Design review of the part built by this model. Coordinates are the model's own, in mm. Face numbers are marked on the shaded views. A direction names the side the tool comes from. Give positions to 0.01 mm unless a question says otherwise; leave off trailing zeros. Write each loop counter-clockwise with the first axis right and the second up, starting at its lowest first coordinate (ties: lowest second). Pieces come first, ordered by that corner, then holes. Notation, with made-up numbers: (4.5, -0.75) -> (52.5, -0.75) arc R26 ccw to (52.5, 24.25) -> close; hole circle Ø2 at (18, -35.5). An arc over 180 degrees is marked (long way). Use CSV: the item, a comma, the result in double quotes.
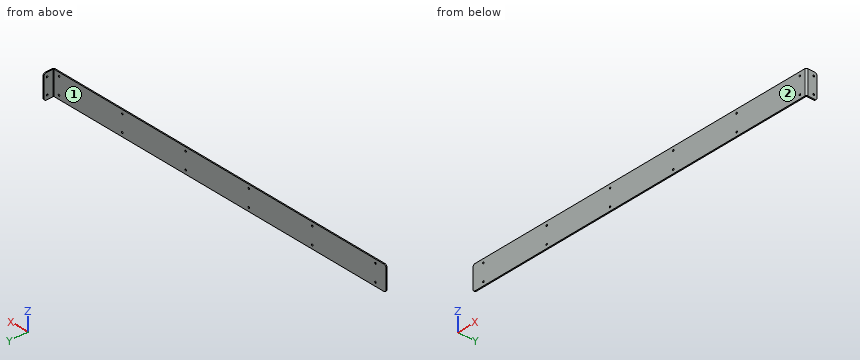
```python
from build123d import *

# Parameters (mm, degrees)
SKETCH1_W                    = 1063.92345
SKETCH1_H                    = 71.4375
BASE_FLANGE1_DEPTH           = 3.2639
EDGE_FLANGE2_DEPTH           = 71.4375
F_10_0_1935_DIAMETER_HOLE1_D = 4.9149
LPATTERN1_COUNT              = 6
LPATTERN1_PITCH              = 202.8825
F_10_0_1935_DIAMETER_HOLE2_D = 4.9149
FILLET1_R                    = 6.35


# Sheet-metal steps are written as plain solids
with BuildPart() as part:
    # Sketch1 → Base-Flange1 (new body)
    with BuildSketch(Plane(origin=(0, 0, 0), x_dir=(1, 0, 0), z_dir=(0, 1, 0))):
        with Locations((-531.961725, 0)):
            Rectangle(SKETCH1_W, SKETCH1_H)
    extrude(amount=-BASE_FLANGE1_DEPTH)

    # Edge-Flange2 section (across the edge) → Edge-Flange2 (add)
    with BuildSketch(Plane(origin=(1.27, 0, 35.71875), x_dir=(-1, 0, 0), z_dir=(0, 0, -1))):
        with BuildLine():
            Line((-3.2639, 1.27), (-3.2639, 28.4861))
            Line((-3.2639, 28.4861), (0, 28.4861))
            Line((0, 28.4861), (0, 1.27))
            ThreePointArc((0, 1.27), (0.371974388, 0.371974388), (1.27, 0))
            Line((1.27, 0), (1.27, -3.2639))
            ThreePointArc((1.27, -3.2639), (-1.935951435, -1.935951435), (-3.2639, 1.27))
        make_face()
    extrude(amount=EDGE_FLANGE2_DEPTH)

    # #10 (0.1935) Diameter Hole1 (through all)
    with Locations(Plane(origin=(0, 0, 0), x_dir=(1, 0, 0), z_dir=(0, 1, 0))):
        with Locations((-16.1036, 24.60625), (-16.1036, -24.60625)):
            f_10_0_1935_diameter_hole1 = Hole(F_10_0_1935_DIAMETER_HOLE1_D / 2)

    # LPattern1: #10 (0.1935) Diameter Hole1 ×6
    with Locations(*[(-i * LPATTERN1_PITCH, 0, 0) for i in range(1, LPATTERN1_COUNT)]):
        add(f_10_0_1935_diameter_hole1, mode=Mode.SUBTRACT)

    # #10 (0.1935) Diameter Hole2 (through all)
    with Locations(Plane.ZY.offset(-1.27)):
        with Locations((-23.8125, 19.05), (23.8125, 19.05)):
            Hole(F_10_0_1935_DIAMETER_HOLE2_D / 2)

    # Fillet1
    fillet1_edges = [part.edges().sort_by_distance(p)[0] for p in [
        (2.90195, 28.4861, 35.71875),
        (2.90195, 28.4861, -35.71875),
        (-1063.92345, -1.63195, -35.71875),
        (-1063.92345, -1.63195, 35.71875),
    ]]
    fillet(fillet1_edges, radius=FILLET1_R)


solid = part.part
```
(1) For line 1 along X through (y, z) = (1.5, -30); line 2 along Y through (x, z) = (-87, 25.5); line 3 along X through (y, z) = (-1.5, 19), list the stretches that pass through material, from the lowest coordinate up. Write a range as [from, to].
Established:
line 1,"x = [1.27, 4.53]"
line 2,"y = [-3.26, 0]"
line 3,"x = [-1063.92, 3.59]"
(2) Clearance check with a flat-ended pin moving along its axis: pin 1 (1.5 mm diameter, centred on x = -134.5, z = 15.5, fed in from +Y). State where the tip first meets the part, or that it passes through.
Established:
pin 1,"stops at y = 0"
(3) Take a section at B-B (y = 9.5). Write out the cut boundary in (x, z).
Established:
outline,"(1.27, -35.72) -> (4.53, -35.72) -> (4.53, 35.72) -> (1.27, 35.72) -> close"
(4) Take a section at A-A (x = -134.5). Write out the cut boundary in (y, z), then the cut area to 3 significant figures.
Established:
outline,"(-3.26, -35.72) -> (0, -35.72) -> (0, 35.72) -> (-3.26, 35.72) -> close"
area,"233 mm2"
(5) Tool access review of the marked faces 1 and 2: name each direction out of +Z, -Z, +X, -X, +Y, -Y from which nothing blocks a thin tool from reaching the whole face with its end or side.
Established:
face 1,"+Z, -Z, -X, +Y"
face 2,"+Z, -Z, +X, -X, -Y"
